Input: part model. Units: mm. Frame: model coordinates. Give positions to 0.01 mm unless a question says otherwise; leave off trailing zeros. Order: outer loops, then holes, each group sorted by start corner. A loop starts at its lowest first (then second) coordinate and runs counter-clockwise, first axis right, second up.
```python
from build123d import *

# Parameters (mm, degrees)
F1_DEPTH = 25.4


with BuildPart() as f1:
    # F0 (on Right) → F1 (new body)
    with BuildSketch(Plane.YZ):
        with BuildLine():
            ThreePointArc((-37.6594869553, -4.7487942502), (-45.0989747132, 13.2117179919), (-63.0594869553, 20.6512057498))
            Line((-63.0594869553, 20.6512057498), (-63.0594869553, 7.9512057498))
            ThreePointArc((-63.0594869553, 7.9512057498), (-54.0792308342, 4.2314618709), (-50.3594869553, -4.7487942502))
            ThreePointArc((-50.3594869553, -4.7487942502), (-54.0792308342, -13.7290503713), (-63.0594869553, -17.4487942502))
            Line((-63.0594869553, -17.4487942502), (-63.0594869553, -30.1487942502))
            ThreePointArc((-63.0594869553, -30.1487942502), (-45.0989747132, -22.7093064923), (-37.6594869553, -4.7487942502))
        make_face()
        with BuildLine():
            Line((394.1405130447, 20.6512057498), (-63.0594869553, 20.6512057498))
            ThreePointArc((-63.0594869553, 20.6512057498), (-45.0989747132, 13.2117179919), (-37.6594869553, -4.7487942502))
            ThreePointArc((-37.6594869553, -4.7487942502), (-45.0989747132, -22.7093064923), (-63.0594869553, -30.1487942502))
            Line((-63.0594869553, -30.1487942502), (394.1405130447, -30.1487942502))
            ThreePointArc((394.1405130447, -30.1487942502), (368.7405130447, -4.7487942502), (394.1405130447, 20.6512057498))
        make_face()
        with BuildLine():
            Line((-63.0594869553, 7.9512057498), (-63.0594869553, 20.6512057498))
            ThreePointArc((-63.0594869553, 20.6512057498), (-88.4594869553, -4.7487942502), (-63.0594869553, -30.1487942502))
            Line((-63.0594869553, -30.1487942502), (-63.0594869553, -17.4487942502))
            ThreePointArc((-63.0594869553, -17.4487942502), (-75.7594869553, -4.7487942502), (-63.0594869553, 7.9512057498))
        make_face()
        with BuildLine():
            ThreePointArc((419.5405130447, -4.7487942502), (412.1010252868, 13.2117179919), (394.1405130447, 20.6512057498))
            Line((394.1405130447, 20.6512057498), (394.1405130447, 7.9512057498))
            ThreePointArc((394.1405130447, 7.9512057498), (403.1207691658, 4.2314618709), (406.8405130447, -4.7487942502))
            ThreePointArc((406.8405130447, -4.7487942502), (403.1207691658, -13.7290503713), (394.1405130447, -17.4487942502))
            Line((394.1405130447, -17.4487942502), (394.1405130447, -30.1487942502))
            ThreePointArc((394.1405130447, -30.1487942502), (412.1010252868, -22.7093064923), (419.5405130447, -4.7487942502))
        make_face()
        with BuildLine():
            Line((394.1405130447, 7.9512057498), (394.1405130447, 20.6512057498))
            ThreePointArc((394.1405130447, 20.6512057498), (368.7405130447, -4.7487942502), (394.1405130447, -30.1487942502))
            Line((394.1405130447, -30.1487942502), (394.1405130447, -17.4487942502))
            ThreePointArc((394.1405130447, -17.4487942502), (381.4405130447, -4.7487942502), (394.1405130447, 7.9512057498))
        make_face()
    extrude(amount=F1_DEPTH)


solid = f1.part
```
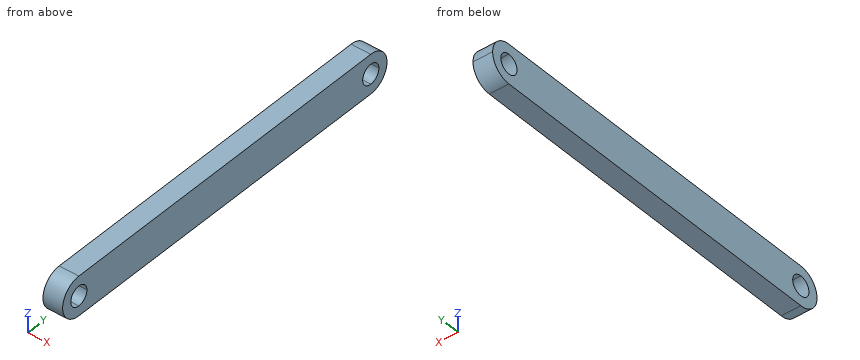
1) First-contact query: P1, Ø1.5, axis at x = 8.5, z = -12.5, coming from the +Y side; P2, Ø8, axis at x = 9.5, z = -15, coming from the +Y side; P3, Ø12, axis at x = 13, z = -15.5, coming from the +Y side. Flat tips, straight axial feed; report the tip coordinate or a pass-through.
2) Cut plane A-A (x = 12.75). Return the cut outline in (y, z).
3) Line query: probe 1 along Y at (x, z) = (6, -4); probe 2 along Y at (x, z) = (3.25, -15); probe 3 along Y at (x, z) = (23.25, 16). Output: solid intervals per line, ascending.
Geometry says:
1. P1: stops at y = 418.56
1. P2: stops at y = 418.76
1. P3: stops at y = 419.09
2. outline: (-63.06, -30.15) - (394.14, -30.15) arc R25.4 ccw to (394.14, 20.65) - (-63.06, 20.65) arc R25.4 ccw to start; hole circle Ø25.4 at (-63.06, -4.75); hole circle Ø25.4 at (394.14, -4.75)
3. probe 1: y = -88.45 to -75.74, -50.38 to 381.46, 406.82 to 419.53
3. probe 2: y = -86.3 to -70.56, -55.56 to 386.64, 401.64 to 417.38
3. probe 3: y = -77.71 to 408.79
